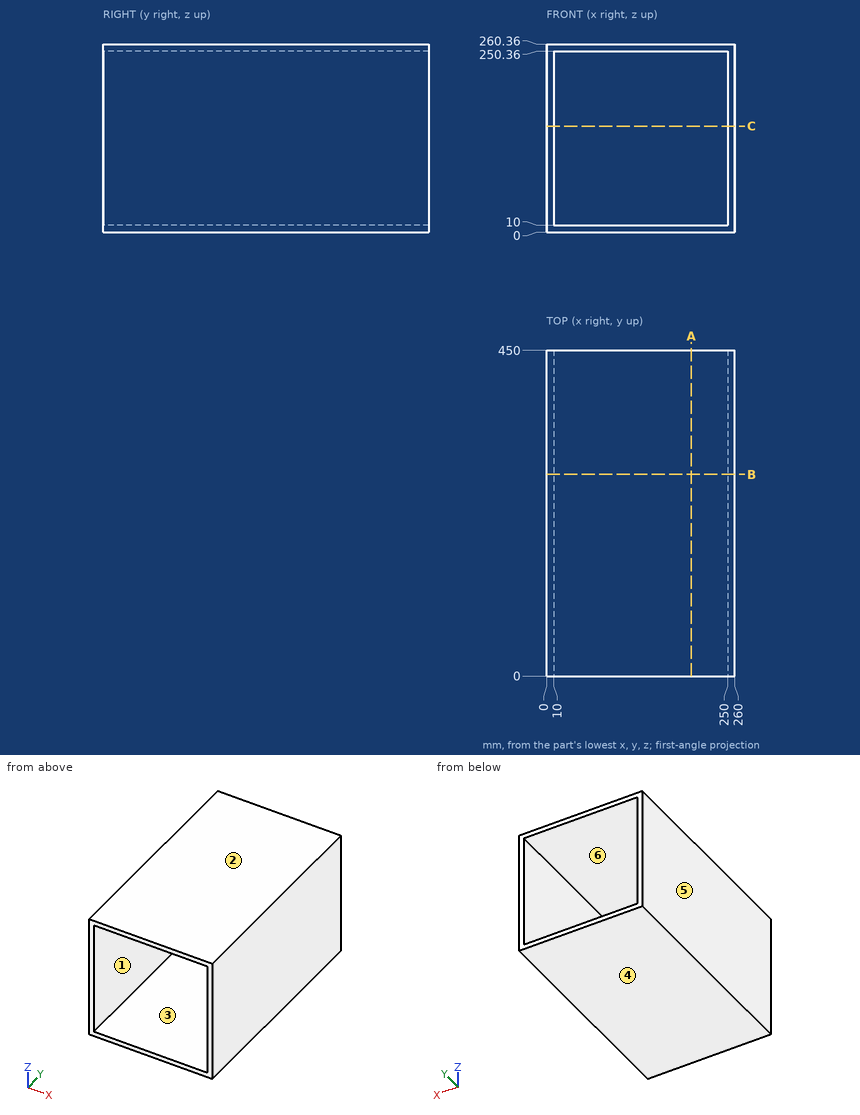
For this review, use the dimensioned drawing (mm, ordinates from the lowest corner) and the shaded views. A direction names the side the tool comes from. Round coordinates to 2 decimals unless told otherwise and drop trailing zeros. Order: outer loops, then holes, each group sorted by start corner. A loop starts at its lowest first (then second) coordinate and runs counter-clockwise, first axis right, second up. Notation, with made-up numbers: (72.25, 14.5) -> (89.25, 14.5) arc R26 ccw to (89.25, 50.5) -> close; hole circle Ø4 at (88.5, -22.5). An arc over 180 degrees is marked (long way). Write item = value, one per line. Start each with the question number.
Item 1: Clearance check with a flat-ended pin moving along its axis: pin 1 Ø3 at (x, y) = (184.5, 388) entering from -Z. State where the tip first meets the part, or that it passes through.
Item 2: Consider section C-C on z = 147. Write out the cut boundary in (x, y).
Item 3: Consider section B-B on y = 278.5. Write out the cut boundary in (x, z), plus the area to 3 significant figures.
Item 4: Consider section A-A on x = 200. Write out the cut boundary in (y, z).
Item 5: For the marked faces 1 and 2, list the 3-axis set-ups (+Z, -Z, +X, -X, +Y, -Y) from which the entire face can be reached by the end or side of a thin tool; tool diameter is ignored.
Item 6: For line 1 along Z through (x, y) = (164, 142.5); line 2 along X through (y, z) = (63, 159.5), list the stretches that pass through material, from the lowest coordinate up.
Item 7: Mouldability with a two-part tool opening along X and no side actions: class the marked faces 3, 4, 5 and 6 as released by +X, released by -X, zero draft, split by the parting line, or undercut.
Conclusion:
q1.pin_1 = 0
q2.outline = (0, 0) -> (10, 0) -> (10, 450) -> (0, 450) -> close; (250, 0) -> (260, 0) -> (260, 450) -> (250, 450) -> close
q3.outline = (0, 0) -> (260, 0) -> (260, 260.36) -> (0, 260.36) -> close; hole (10, 10) -> (250, 10) -> (250, 250.36) -> (10, 250.36) -> close
q3.area = 10,000 mm2
q4.outline = (0, 0) -> (450, 0) -> (450, 10) -> (0, 10) -> close; (0, 250.36) -> (450, 250.36) -> (450, 260.36) -> (0, 260.36) -> close
q5.face_1 = +Y, -Y
q5.face_2 = +Z, +X, -X, +Y, -Y
q6.line_1 = 0 to 10, 250.36 to 260.36
q6.line_2 = 0 to 10, 250 to 260
q7.face_3 = undercut
q7.face_4 = zero draft
q7.face_5 = released by -X
q7.face_6 = undercut
